Could you check a few things on this model? Use its own coordinates, in mm. A direction names the side the tool comes from. Coordinates: 2 decimals unless noted, no trailing zeros. Loops run counter-clockwise (first coordinate to the right, second up) from the corner with the lowest first, then second, coordinate; pieces in that order, holes last. Notation, with made-up numbers: M 12.5,35.5 L 17.5,35.5 A13 ccw 17.5,39.5 Z; hole C 80,58.5 d11. An arc over 180 degrees is marked long. Use one line per item in the form item = value. Start each with the question number.
```python
from build123d import *

# Parameters (mm, degrees)
F1_DEPTH = 50
F2_W     = 40
F2_H     = 10
F3_DEPTH = 30
F2_W_2   = 150
F4_DEPTH = 10
F5_DEPTH = 20


# Not quite as in the source:
# - a pattern or mirror of a feature is missing from the dataset's text; its kind, count and spacing are read off the source's solid


with BuildPart() as f1:
    # F0 (on Top) → F1 (new body)
    with BuildSketch(Plane.XY):
        with BuildLine():
            Line((-35, -25), (-35, -40))
            Line((-35, -40), (115, -40))
            Line((115, -40), (115, 40))
            Line((115, 40), (-35, 40))
            Line((-35, 40), (-35, 25))
            Line((-35, 25), (0, 25))
            ThreePointArc((0, 25), (25, 0), (0, -25))
            Line((0, -25), (-35, -25))
        make_face()
    extrude(amount=F1_DEPTH)

    # F2 (on face) → F3 (cut)
    with BuildSketch(Plane.XZ.offset(40)):
        with Locations((-15, 45)):
            Rectangle(F2_W, F2_H)
        Polygon((115, 50), (55, 50), (91, 35), (115, 25), align=None)
    f3 = extrude(amount=-F3_DEPTH, mode=Mode.SUBTRACT)

    # F3_copies: F3 across plane
    add(f3.mirror(Plane.ZX), mode=Mode.SUBTRACT)

    # F2 (on face) → F4 (cut)
    with BuildSketch(Plane.XZ.offset(40)):
        with Locations((40, 15)):
            Rectangle(F2_W_2, F2_H)
    f4 = extrude(amount=-F4_DEPTH, mode=Mode.SUBTRACT)

    # F4_copies: F4 across plane
    add(f4.mirror(Plane.ZX), mode=Mode.SUBTRACT)

    # F2 (on face) → F5 (cut)
    with BuildSketch(Plane.XZ.offset(40)):
        with BuildLine():
            Line((55, 50), (25, 50))
            ThreePointArc((25, 50), (29.3933982822, 39.3933982822), (40, 35))
            Line((40, 35), (91, 35))
            Line((91, 35), (55, 50))
        make_face()
    f5 = extrude(amount=-F5_DEPTH, mode=Mode.SUBTRACT)

    # F5_copies: F5 across plane
    add(f5.mirror(Plane.ZX), mode=Mode.SUBTRACT)


solid = f1.part
```
Item 1: Please list where these lines run through material, in increasing order: line 1 along Y through (x, z) = (-14, 31); line 2 along Z through (x, y) = (-23.5, 33); line 3 along Z through (x, y) = (39, -37).
Item 2: For faces 5 (the flat face through (98, -10, 43)), 6 (the flat face through (47, 1, 50)), 7 (the flat face through (-15, 32, 40)), 8 (the flat face through (50, 20, 43)), which set-ups out of +Z, -Z, +X, -X, +Y, -Y let a thin tool reach every point of the face, with its end or its side?
Item 3: I want a section at B-B (x = 45). Write out the boundary of the cut face in (y, z).
Item 4: I want a section at D-D (z = 14.5). Write out the boundary of the cut face in (x, y).
Item 5: I want a section at A-A (z = 27). Write out the boundary of the cut face in (x, y), plus the area to 3 significant figures.
Item 6: I want a section at C-C (y = 0). Write out the boundary of the cut face in (x, z), plus the area to 3 significant figures.
Item 7: I'm going to push flat-ended pins straight in: P1, Ø11, axis at y = 35, z = 47.5, coming from the -X side; P2, Ø8, axis at x = 33, y = 36.5, coming from the -Z side; P3, Ø1.5, axis at y = 9, z = 26.5, coming from the -X side; P4, Ø5, axis at y = 3, z = 6, coming from the -X side. Where does each tip first touch, or does it pass through?
Item 8: Thinking about a two-plate mould opening in Z: for faces 1 (the flat face through (98, 10, 43)), 2 (the flat face through (39, -35, 10)), 3 (the flat face through (56, 1, 0)), 4 (the flat face through (39, 35, 20)), which applies, pulls with the +Z half, pulls with the -Z half, needs draft (parallel to the pull), parting line crosses it, or undercut?
Worked answers:
q1.line_1 = -40 to -25, 25 to 40
q1.line_2 = 0 to 10, 20 to 40
q1.line_3 = 0 to 10, 20 to 35.03
q2.face_5 = +Z, +X, -Y
q2.face_6 = +Z, +X, -X, +Y, -Y
q2.face_7 = +Z, -X, +Y, -Y
q2.face_8 = +Z, +X, +Y
q3.outline = M -40,0 L 40,0 L 40,10 L 30,10 L 30,20 L 40,20 L 40,35 L 20,35 L 20,50 L -20,50 L -20,35 L -40,35 L -40,20 L -30,20 L -30,10 L -40,10 Z
q4.outline = M -35,-30 L 115,-30 L 115,30 L -35,30 L -35,25 L 0,25 A25 cw 0,-25 L -35,-25 Z
q5.outline = M -35,-40 L 110.2,-40 L 110.2,-10 L 115,-10 L 115,10 L 110.2,10 L 110.2,40 L -35,40 L -35,25 L 0,25 A25 cw 0,-25 L -35,-25 Z
q5.area = 8,980 mm²
q6.outline = M 25,0 L 115,0 L 115,50 L 25,50 Z
q6.area = 4,500 mm²
q7.P1 = 5
q7.P2 = 0
q7.P3 = 23.02
q7.P4 = 24.39
q8.face_1 = needs draft
q8.face_2 = undercut
q8.face_3 = pulls with the -Z half
q8.face_4 = undercut
